Part model, mm, in its own coordinate system. A direction names the side the tool comes from. Round coordinates to 2 decimals unless told otherwise and drop trailing zeros. Loops run counter-clockwise (first coordinate to the right, second up) from the corner with the lowest first, then second, coordinate; pieces in that order, holes last. Notation, with made-up numbers: (25.25, 36.5) - (34.25, 36.5) arc R22 cw to (34.25, 53.5) - close; hole circle Ø7 at (12.5, 49.5). An arc over 180 degrees is marked (long way). Put each result on its own line as item: value.
Autodesk Inventor part; units mm, degrees
ref_plane "YZ Plane" through (0, 0, 0) normal (1, 0, 0) x (0, 1, 0)
ref_plane "XZ Plane" through (0, 0, 0) normal (0, 1, 0) x (-1, 0, 0)
ref_plane "XY Plane" through (0, 0, 0) normal (0, 0, 1) x (1, 0, 0)
sketch "Skizze1" plane through (0, 0, 0) normal (0, 1, 0) x (-1, 0, 0)
  arc A0 (-1, 30.4836) -> (-30.5, 0) centre (0, 0) ccw
  arc A1 (-6.2857, 34.431) -> (-35, 0) centre (0, 0) ccw
  line L0 (-1, 45) -> (-5.9982, 45.1342)
  line L1 (-5.9982, 45.1342) -> (-6.2857, 34.431)
  line L2 (0, 0) -> (-14.1914, 0) construction
  line L3 (-1, 30.4836) -> (-1, 45)
  arc A2 (-30.5, 0) -> (-1, -30.4836) centre (0, 0) ccw
  arc A3 (-35, 0) -> (-6.2857, -34.431) centre (0, 0) ccw
  line L4 (-1, -45) -> (-5.9982, -45.1342)
  line L5 (-5.9982, -45.1342) -> (-6.2857, -34.431)
  line L6 (-1, -30.4836) -> (-1, -45)
  dimension "d59" = 30.5
  dimension "d60" = 35
  dimension "d72" = 1
  dimension "d73" = 5
  dimension "d74" = 45
  dimension "d75" = 10.7071
extrude "Extrusion1" add sketch "Skizze1" along normal blind 20
ref_plane "Arbeitsebene1" through (35, 20, 0) normal (1, 0, 0) x (0, 1, 0)
sketch "Skizze3" plane through (35, 20, 0) normal (1, 0, 0) x (0, 1, 0)
  line L0 (0, -30.4836) -> (0, 30.4836)
  line L1 (0, 20) -> (-20, 20)
  line L2 (-20, 20) -> (-20, -20)
  line L3 (-20, -20) -> (0, -20)
  line L4 (0, -20) -> (0, 20)
  point P0 (-20, 0)
  dimension "d28" = 20
  dimension "d30" = 20
  dimension "d31" = 20
extrude "Extrusion2" add sketch "Skizze3" against normal blind 10 and the other way blind 2
sketch "Skizze5" plane through (1, 0, 30.4836) normal (-1, 0, 0) x (0, 0, 1)
  line L0 (14.5, 0) -> (14.5, 20) construction
  line L1 (14.5, 10) -> (-75.5, 10) construction
  line L2 (-75.5, 0) -> (-75.5, 20) construction
  line L3 (-75.5, 20) -> (-61, 20) construction
  line L4 (-68.25, 20) -> (-68.25, 0) construction
  line L5 (-61, 0) -> (-75.5, 0) construction
  line L6 (0, 20) -> (14.5, 20) construction
  line L7 (7.25, 20) -> (7.25, 0) construction
  line L8 (14.5, 0) -> (0, 0) construction
  point P0 (-30.5, 0)
  point P1 (7.25, 10)
  point P2 (-68.25, 10)
hole "Bohrung3" at (1, 10, 37.7336) at (1, 10, -37.7664) direction (1, 0, 0) diameter 3.3 end through all
ref_plane "Arbeitsebene2" through (23, 20, 0) normal (1, 0, 0) x (0, 1, 0)
sketch "Skizze7" plane through (23, 20, 0) normal (1, 0, 0) x (0, 1, 0)
  line L0 (0, 30.4836) -> (0, -30.4836)
  point P0 (-20, 0)
  point P1 (-10, 15)
  point P2 (-10, -15)
  dimension "d81" = 10
  dimension "d82" = 10
  dimension "d84" = 15
  dimension "d94" = 15
hole "Bohrung4" at (23, 10, 15) at (23, 10, -15) direction (1, 0, 0) diameter 4.3 end through all counterbore diameter 8 counterbore depth 8
delete faces "Fläche löschen1" heal yes whole lump no faces at (25, 2.4288, 4.0204)
properties part number "spannringe"
1. Band-saw the part on A-A (z = 15). List the corners of the cut face in (x, y).
A:
outline: (26.56, 0) - (37, 0) - (37, 7.85) - (31, 7.85) - (31, 6) - (26.56, 6) - close; (26.56, 14) - (31, 14) - (31, 12.15) - (37, 12.15) - (37, 20) - (26.56, 20) - close
2. Band-saw the part on C-C (y = 16). List the corners of the cut face in (x, z).
A:
outline: (1, -45) - (6, -45.13) - (6.29, -34.43) arc R35 ccw to (28.72, -20) - (37, -20) - (37, 20) - (28.72, 20) arc R35 ccw to (6.29, 34.43) - (6, 45.13) - (1, 45) - (1, 30.48) arc R30.5 cw to (30.5, 0) arc R30.5 cw to (1, -30.48) - close
3. Band-saw the part on D-D (y = 10). Give the number of separate pieces and of enclosed holes in the cut face, plus the area to 3 significant figures.
A:
separate pieces: 5
enclosed holes: 0
area: 561 mm²
4. Probe line 1 along Y through (x, z) = (26.75, 15); line 2 along Z through (x, y) = (35, 10); line 3 along Y through (x, z) = (34, 15). List the from-to ranges inside material, lowest first. Write a range as [from, to].
A:
line 1: y = [0, 6], [14, 20]
line 2: z = [-20, -17.15], [-12.85, 12.85], [17.15, 20]
line 3: y = [0, 7.85], [12.15, 20]
5. Pin check, flat tips, straight feed: P1, Ø4.5, axis at y = 10, z = 37.73, coming from the -X side; P2, Ø4, axis at x = 34, y = 7, coming from the +Z side; P3, Ø6.5, axis at x = 33.5, y = 14, coming from the -Z side; P4, Ø2.5, axis at y = 10.5, z = -17, coming from the -X side. Stop position of each tip, or through.
A:
P1: stops at x = 1
P2: stops at z = 20
P3: stops at z = -20
P4: stops at x = 31
6. Two-plate mould, pull along Z, no slides. Class faces 1 (the cylindrical face through (19.094, 9.86, 29.333)), 2 (the cylindrical face through (3.657, 9.927, -39.415)), 3 (the flat face through (31, 0, 0)): pulls with the +Z half, pulls with the -Z half, needs draft (parallel to the pull), parting line crosses it, or undercut.
A:
face 1: pulls with the +Z half
face 2: undercut
face 3: needs draft
7. Tool access for faces 4 (the flat face through (31, 12, 17)), 5 (the flat face through (1, 12, 38)), 6 (the flat face through (33, 10, -20)), 7 (the flat face through (33, 10, 20)): list every direction of +Z, -Z, +X, -X, +Y, -Y with a clear straight run to the whole face (end or side of a thin tool).
A:
face 4: -X
face 5: +Z, -Z, -X, +Y, -Y
face 6: -Z, +X, +Y, -Y
face 7: +Z, +X, +Y, -Y
8. Band-saw the part on B-B (x = 20). List the corners of the cut face in (y, z).
A:
outline: (0, -28.72) - (20, -28.72) - (20, -23.03) - (0, -23.03) - close; (0, 23.03) - (20, 23.03) - (20, 28.72) - (0, 28.72) - close
